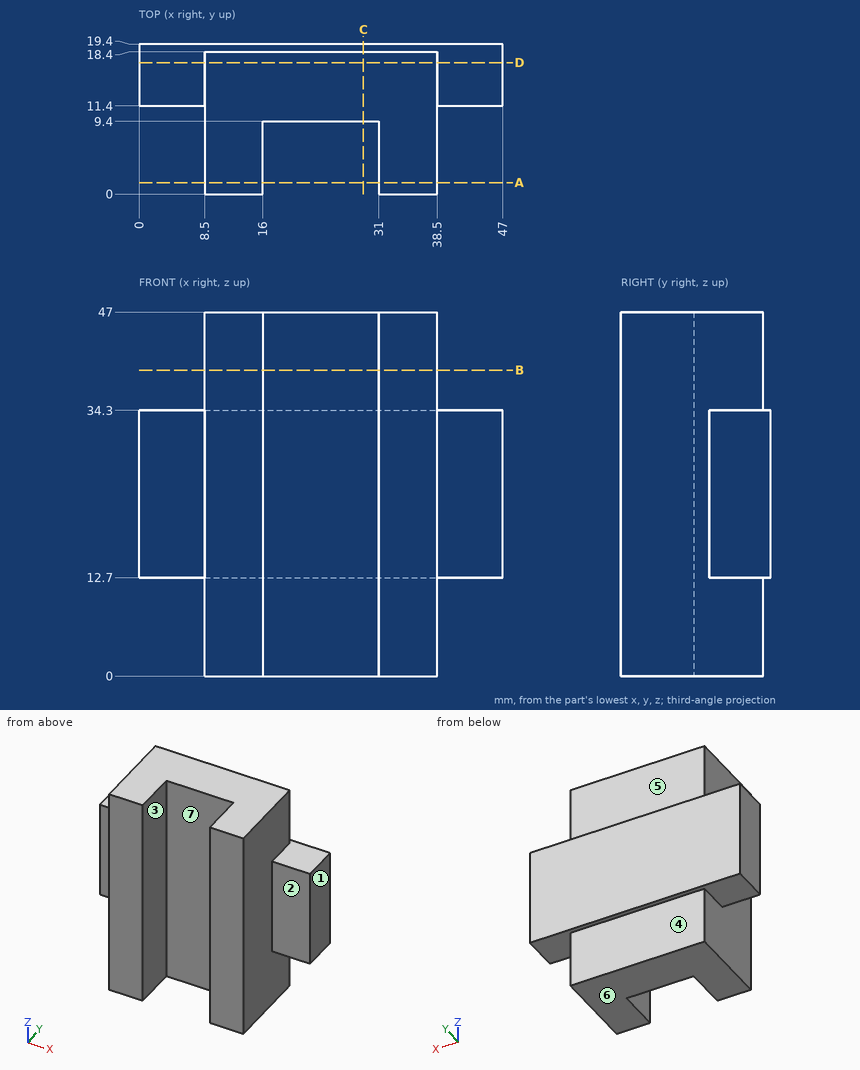
Job drawing, mm, ordinate dimensions from the low corner. One solid piece. A direction names the side the tool comes from. Round coordinates to 2 decimals unless told otherwise and drop trailing zeros. Loops run counter-clockwise (first coordinate to the right, second up) from the corner with the lowest first, then second, coordinate; pieces in that order, holes last.
Item 1: Cut at D-D, the plane y = 17. Give the cut face in (x, z).
Item 2: Drill centre lines: line 1 (X direction, y = 5.5, z = 39); line 2 (Z direction, x = 4, y = 12); line 3 (Y direction, x = 29, z = 44). Where is each one in solid material? Low to high.
Item 3: Cut at B-B, the plane z = 39.5. Give the cut face in (x, y), then the cut area to 3 significant figures.
Item 4: Cut at A-A, the plane y = 1.5. Give the cut face in (x, z).
Item 5: Drop flat-ended pins along their axis: P1, Ø6, axis at y = 3.5, z = 31.5, coming from the +X side; P2, Ø5.5, axis at y = 10.5, z = 16, coming from the +X side; P3, Ø7, axis at x = 42.5, z = 28.5, coming from the -Y side; P4, Ø6.5, axis at x = 18, z = 4, coming from the +Y side. Give the stop position or say it passes through.
Item 6: Mould opens along X. For the marked faces 1, 2 and 3 say: +X half, -X half, draft (parallel to the pull), parting line (faces both ways), or undercut.
Item 7: 3-axis set-ups, long thin cutter, end or side, ignore diameter. For the marked faces 4, 5, 6 and 7: which of +Z, -Z, +X, -X, +Y, -Y reach the whole face in a straight line?
Item 8: Cut at C-C, the plane x = 29. Give the cut face in (y, z), then the cut area to 3 significant figures.
A:
1. outline: (0, 12.7) - (8.5, 12.7) - (8.5, 0) - (38.5, 0) - (38.5, 12.7) - (47, 12.7) - (47, 34.3) - (38.5, 34.3) - (38.5, 47) - (8.5, 47) - (8.5, 34.3) - (0, 34.3) - close
2. line 1: x = 8.5 to 16, 31 to 38.5
2. line 2: z = 12.7 to 34.3
2. line 3: y = 9.4 to 18.4
3. outline: (8.5, 0) - (16, 0) - (16, 9.4) - (31, 9.4) - (31, 0) - (38.5, 0) - (38.5, 18.4) - (8.5, 18.4) - close
3. area: 411 mm2
4. outline: (8.5, 0) - (16, 0) - (16, 47) - (8.5, 47) - close; (31, 0) - (38.5, 0) - (38.5, 47) - (31, 47) - close
5. P1: stops at x = 38.5
5. P2: stops at x = 47
5. P3: stops at y = 11.4
5. P4: stops at y = 18.4
6. face 1: +X half
6. face 2: draft
6. face 3: undercut
7. face 4: -Z, +X, -X, +Y
7. face 5: +Z, +X, -X, +Y
7. face 6: -Z, +X, -X, +Y, -Y
7. face 7: +Z, -Z, -Y
8. outline: (9.4, 0) - (18.4, 0) - (18.4, 12.7) - (19.4, 12.7) - (19.4, 34.3) - (18.4, 34.3) - (18.4, 47) - (9.4, 47) - close
8. area: 445 mm2
